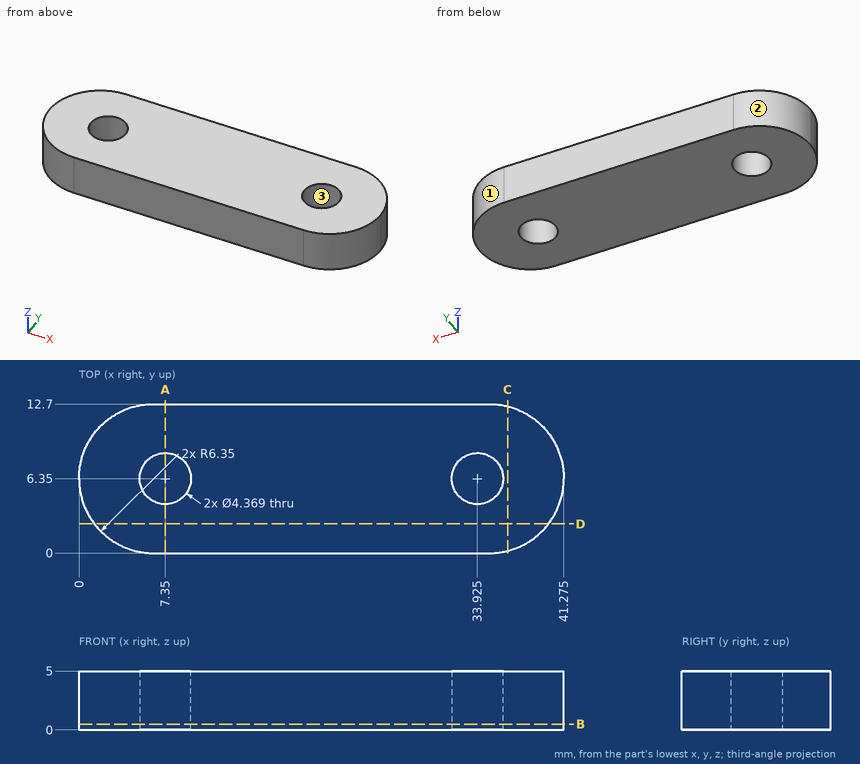
The figure shows three views and two pictorial views of one solid part (mm, origin at its lowest corner). Answer the questions. Give positions to 0.01 mm unless a question says otherwise; leave off trailing zeros. Order: outer loops, then holes, each group sorted by start corner. A loop starts at its lowest first (then second) coordinate and runs counter-clockwise, first axis right, second up. Notation, with made-up numbers: (34, 38.25) -> (51, 38.25) arc R23 cw to (51, 58.25) -> close; hole circle Ø10 at (55, 29.5). An arc over 180 degrees is marked (long way). Answer as a JSON object with one key per item and string values. Group by question number.
Item 1: The part is cut by section A-A on x = 7.35. Write down the section's boundary in (y, z).
Item 2: Consider L1, parallel to X at y = 6.25, z = 2.85; L2, parallel to X at y = 4.5, z = 2.85 (1 decimal); L3, parallel to Y at x = 38, z = 0.7 (1 decimal). Determine where each line is inside the solid, lowest interval first. Write a range as from..to.
Item 3: The part is cut by section C-C on x = 36.5. Write down the section's boundary in (y, z), and give its area (3 significant figures).
Item 4: Determine the mould class of the marked faces 1, 2 and 3 for opening direction X: pulls with the +X half, pulls with the -X half, needs draft (parallel to the pull), parting line crosses it, or undercut.
Item 5: The part is cut by section B-B on z = 0.5. Give the number of separate pieces and of enclosed holes in the cut face, and give its area (3 significant figures).
Item 6: Flat-ended cylindrical pins translate along their axes: pin 1 (4 mm diameter, centred on x = 33.925, y = 6.35, fed in from -Z); pin 2 (2 mm diameter, centred on y = 4.5, z = 3.5, fed in from -X). Find the tip coordinate at first contact, or state that the pin passes through.
Item 7: The part is cut by section D-D on y = 2.5. Write down the section's boundary in (x, z) (1 decimal).
Result set:
{
 "1": {"outline": "(0, 0) -> (4.17, 0) -> (4.17, 5) -> (0, 5) -> close; (8.53, 0) -> (12.7, 0) -> (12.7, 5) -> (8.53, 5) -> close"},
 "2": {"L1": "0..5.17, 9.53..31.74, 36.11..41.27", "L2": "0.3..6.2, 8.5..32.8, 35.1..41", "L3": "0.8..11.9"},
 "3": {"outline": "(0.2, 0) -> (12.5, 0) -> (12.5, 5) -> (0.2, 5) -> close", "area": "61.5 mm²"},
 "4": {"face 1": "pulls with the +X half", "face 2": "pulls with the -X half", "face 3": "undercut"},
 "5": {"separate pieces": "1", "enclosed holes": "2", "area": "460 mm²"},
 "6": {"pin 1": "through", "pin 2": "x = 0.06"},
 "7": {"outline": "(1.3, 0) -> (40, 0) -> (40, 5) -> (1.3, 5) -> close"}
}
